```python
from build123d import *

# Parameters (mm, degrees)
SKETCH_1_R      = 3
SKETCH_1_R_2    = 2.05
EXTRUDE_2_DEPTH = 2
FILLET_1_R      = 1.3


with BuildPart() as part:
    # 草图1 → 凸台-拉伸2 (new body)
    with BuildSketch(Plane.XY):
        with BuildLine():
            Line((-55.962487977, 23.496493589), (-55.962487977, 8.046493589))
            Line((-55.962487977, 8.046493589), (-51.962487977, 8.046493589))
            Line((-51.962487977, 8.046493589), (-51.962487977, 9.496493589))
            Line((-51.962487977, 9.496493589), (-48.762487977, 9.496493589))
            Line((-48.762487977, 9.496493589), (-48.762487977, 8.046493589))
            Line((-48.762487977, 8.046493589), (-45.562487977, 8.046493589))
            Line((-45.562487977, 8.046493589), (-45.562487977, 3.946493589))
            Line((-45.562487977, 3.946493589), (-48.762487977, 3.946493589))
            Line((-48.762487977, 3.946493589), (-48.762487977, 2.496493589))
            Line((-48.762487977, 2.496493589), (-51.962487977, 2.496493589))
            Line((-51.962487977, 2.496493589), (-51.962487977, 3.946493589))
            Line((-51.962487977, 3.946493589), (-55.962487977, 3.946493589))
            Line((-55.962487977, 3.946493589), (-55.962487977, -5.003506411))
            Line((-55.962487977, -5.003506411), (-60.962487977, -5.003506411))
            Line((-60.962487977, -5.003506411), (-60.962487977, -13.003506411))
            Line((-60.962487977, -13.003506411), (-55.962487977, -13.003506411))
            Line((-55.962487977, -13.003506411), (-55.962487977, -21.953506411))
            Line((-55.962487977, -21.953506411), (-51.962487977, -21.953506411))
            Line((-51.962487977, -21.953506411), (-51.962487977, -20.503506411))
            Line((-51.962487977, -20.503506411), (-48.762487977, -20.503506411))
            Line((-48.762487977, -20.503506411), (-48.762487977, -21.953506411))
            Line((-48.762487977, -21.953506411), (-45.562487977, -21.953506411))
            Line((-45.562487977, -21.953506411), (-45.562487977, -26.053506411))
            Line((-45.562487977, -26.053506411), (-48.762487977, -26.053506411))
            Line((-48.762487977, -26.053506411), (-48.762487977, -27.503506411))
            Line((-48.762487977, -27.503506411), (-51.962487977, -27.503506411))
            Line((-51.962487977, -27.503506411), (-51.962487977, -26.053506411))
            Line((-51.962487977, -26.053506411), (-55.962487977, -26.053506411))
            Line((-55.962487977, -26.053506411), (-55.962487977, -35.003506411))
            Line((-55.962487977, -35.003506411), (-60.962487977, -35.003506411))
            Line((-60.962487977, -35.003506411), (-60.962487977, -43.003506411))
            Line((-60.962487977, -43.003506411), (-55.962487977, -43.003506411))
            Line((-55.962487977, -43.003506411), (-55.962487977, -51.953506411))
            Line((-55.962487977, -51.953506411), (-51.962487977, -51.953506411))
            Line((-51.962487977, -51.953506411), (-51.962487977, -50.503506411))
            Line((-51.962487977, -50.503506411), (-48.762487977, -50.503506411))
            Line((-48.762487977, -50.503506411), (-48.762487977, -51.953506411))
            Line((-48.762487977, -51.953506411), (-45.562487977, -51.953506411))
            Line((-45.562487977, -51.953506411), (-45.562487977, -56.053506411))
            Line((-45.562487977, -56.053506411), (-48.762487977, -56.053506411))
            Line((-48.762487977, -56.053506411), (-48.762487977, -57.503506411))
            Line((-48.762487977, -57.503506411), (-51.962487977, -57.503506411))
            Line((-51.962487977, -57.503506411), (-51.962487977, -56.053506411))
            Line((-51.962487977, -56.053506411), (-55.962487977, -56.053506411))
            Line((-55.962487977, -56.053506411), (-55.962487977, -61.503506411))
            Line((-55.962487977, -61.503506411), (-67.962487977, -61.503506411))
            Line((-67.962487977, -61.503506411), (-67.962487977, -65.791888255))
            Line((-67.962487977, -65.791888255), (38.037512023, -65.791888255))
            Line((38.037512023, -65.791888255), (38.037512023, -61.503506411))
            Line((38.037512023, -61.503506411), (26.037512023, -61.503506411))
            Line((26.037512023, -61.503506411), (26.037512023, -56.053506411))
            Line((26.037512023, -56.053506411), (22.037512023, -56.053506411))
            Line((22.037512023, -56.053506411), (22.037512023, -57.503506411))
            Line((22.037512023, -57.503506411), (18.837512023, -57.503506411))
            Line((18.837512023, -57.503506411), (18.837512023, -56.053506411))
            Line((18.837512023, -56.053506411), (15.637512023, -56.053506411))
            Line((15.637512023, -56.053506411), (15.637512023, -51.953506411))
            Line((15.637512023, -51.953506411), (18.837512023, -51.953506411))
            Line((18.837512023, -51.953506411), (18.837512023, -50.503506411))
            Line((18.837512023, -50.503506411), (22.037512023, -50.503506411))
            Line((22.037512023, -50.503506411), (22.037512023, -51.953506411))
            Line((22.037512023, -51.953506411), (26.037512023, -51.953506411))
            Line((26.037512023, -51.953506411), (26.037512023, -43.003506411))
            Line((26.037512023, -43.003506411), (31.037512023, -43.003506411))
            Line((31.037512023, -43.003506411), (31.037512023, -35.003506411))
            Line((31.037512023, -35.003506411), (26.037512023, -35.003506411))
            Line((26.037512023, -35.003506411), (26.037512023, -26.053506411))
            Line((26.037512023, -26.053506411), (22.037512023, -26.053506411))
            Line((22.037512023, -26.053506411), (22.037512023, -27.503506411))
            Line((22.037512023, -27.503506411), (18.837512023, -27.503506411))
            Line((18.837512023, -27.503506411), (18.837512023, -26.053506411))
            Line((18.837512023, -26.053506411), (15.637512023, -26.053506411))
            Line((15.637512023, -26.053506411), (15.637512023, -21.953506411))
            Line((15.637512023, -21.953506411), (18.837512023, -21.953506411))
            Line((18.837512023, -21.953506411), (18.837512023, -20.503506411))
            Line((18.837512023, -20.503506411), (22.037512023, -20.503506411))
            Line((22.037512023, -20.503506411), (22.037512023, -21.953506411))
            Line((22.037512023, -21.953506411), (26.037512023, -21.953506411))
            Line((26.037512023, -21.953506411), (26.037512023, -13.003506411))
            Line((26.037512023, -13.003506411), (31.037512023, -13.003506411))
            Line((31.037512023, -13.003506411), (31.037512023, -5.003506411))
            Line((31.037512023, -5.003506411), (26.037512023, -5.003506411))
            Line((26.037512023, -5.003506411), (26.037512023, 3.946493589))
            Line((26.037512023, 3.946493589), (22.037512023, 3.946493589))
            Line((22.037512023, 3.946493589), (22.037512023, 2.496493589))
            Line((22.037512023, 2.496493589), (18.837512023, 2.496493589))
            Line((18.837512023, 2.496493589), (18.837512023, 3.946493589))
            Line((18.837512023, 3.946493589), (15.637512023, 3.946493589))
            Line((15.637512023, 3.946493589), (15.637512023, 8.046493589))
            Line((15.637512023, 8.046493589), (18.837512023, 8.046493589))
            Line((18.837512023, 8.046493589), (18.837512023, 9.496493589))
            Line((18.837512023, 9.496493589), (22.037512023, 9.496493589))
            Line((22.037512023, 9.496493589), (22.037512023, 8.046493589))
            Line((22.037512023, 8.046493589), (26.037512023, 8.046493589))
            Line((26.037512023, 8.046493589), (26.037512023, 23.496493589))
            Line((26.037512023, 23.496493589), (26.037512023, 31.722989041))
            ThreePointArc((26.037512023, 31.722989041), (-14.962487977, 51.269592797), (-55.962487977, 31.722989041))
            Line((-55.962487977, 31.722989041), (-55.962487977, 23.496493589))
        make_face()
        with Locations((-14.962487977, -25.253506411)):
            Circle(SKETCH_1_R, mode=Mode.SUBTRACT)
        with Locations((4.523083608, -12.753506411)):
            Circle(SKETCH_1_R, mode=Mode.SUBTRACT)
        with Locations((-14.962487977, -1.503506411)):
            Circle(SKETCH_1_R_2, mode=Mode.SUBTRACT)
        with Locations((-35.530591317, 10.371493589)):
            Circle(SKETCH_1_R, mode=Mode.SUBTRACT)
        with Locations((-34.448059562, -12.753506411)):
            Circle(SKETCH_1_R, mode=Mode.SUBTRACT)
        with Locations((5.605615363, 10.371493589)):
            Circle(SKETCH_1_R, mode=Mode.SUBTRACT)
        with Locations((-14.962487977, 20.996493589)):
            Circle(SKETCH_1_R, mode=Mode.SUBTRACT)
        with Locations((18.271530739, -34.737525127)):
            Circle(SKETCH_1_R_2, mode=Mode.SUBTRACT)
        with Locations((-14.962487977, -48.503506411)):
            Circle(SKETCH_1_R_2, mode=Mode.SUBTRACT)
        with Locations((-48.196506692, -34.737525127)):
            Circle(SKETCH_1_R_2, mode=Mode.SUBTRACT)
        with Locations((-48.196506692, 31.730512305)):
            Circle(SKETCH_1_R_2, mode=Mode.SUBTRACT)
        with Locations((-14.962487977, 45.496493589)):
            Circle(SKETCH_1_R_2, mode=Mode.SUBTRACT)
        with Locations((18.271530739, 31.730512305)):
            Circle(SKETCH_1_R_2, mode=Mode.SUBTRACT)
    extrude(amount=EXTRUDE_2_DEPTH)

    # 圆角1
    fillet_1_edges = [part.edges().sort_by_distance(p)[0] for p in [
        (-60.962487977, -43.003506411, 1),
        (-60.962487977, -35.003506411, 1),
        (-60.962487977, -13.003506411, 1),
        (-60.962487977, -5.003506411, 1),
        (31.037512023, -5.003506411, 1),
        (31.037512023, -13.003506411, 1),
        (31.037512023, -35.003506411, 1),
        (31.037512023, -43.003506411, 1),
    ]]
    fillet(fillet_1_edges, radius=FILLET_1_R)


solid = part.part
```
Verification items for the finished model (mm, model axes). Coordinates: 2 decimals unless noted, no trailing zeros. Order: outer loops, then holes, each group sorted by start corner. A loop starts at its lowest first (then second) coordinate and runs counter-clockwise, first axis right, second up. Notation, with made-up numbers: (35.25, -26.5) -> (94.25, -26.5) arc R11 ccw to (94.25, -15.5) -> close; hole circle Ø11 at (17, 89.5). An arc over 180 degrees is marked (long way). Put each result on its own line as item: value. Start each with the question number.
1) Go/stop test with a flat-tipped pin: pin 1 (1 mm diameter, centred on y = -1, z = 1, fed in from +X). Record where the tip stops, or that it passes through.
2) Cross-section at C-C (y = 40). Enter the section's corners in (x, z).
3) Cross-section at A-A (z = 1.6). State how many separate pieces and enclosed holes the cut face has, plus the area to 3 significant figures.
4) Cross-section at B-B (x = -1). Enter the section's corners in (y, z).
5) Release check for a two-part mould opening along X. For faces 1 (the flat face through (-16, -6, 0)), 2 (the cylindrical face through (-14.305, 51.265, 0.986)), 3 (the cylindrical face through (-38.528, 10.503, 0.986)) record: pulls with the +X half, pulls with the -X half, needs draft (parallel to the pull), parting line crosses it, or undercut.
6) Material ranges on L1, parallel to X at y = -51.5, z = 1.6; L2, parallel to Y at x = -12.5, z = 1.7; L3, parallel to Y at x = 31.5, z = 1.95, recorded low to high.
Geometry check:
1. pin 1: stops at x = 26.04
2. outline: (-47.56, 0) -> (17.63, 0) -> (17.63, 2) -> (-47.56, 2) -> close
3. separate pieces: 1
3. enclosed holes: 13
3. area: 8,800 mm^2
4. outline: (-65.79, 0) -> (49.39, 0) -> (49.39, 2) -> (-65.79, 2) -> close
5. face 1: needs draft
5. face 2: parting line crosses it
5. face 3: undercut
6. L1: x = -55.96 to -51.96, -48.76 to 18.84, 22.04 to 26.04
6. L2: y = -65.79 to -26.97, -23.54 to 19.28, 22.71 to 51.21
6. L3: y = -65.79 to -61.5
